```python
from build123d import *

# Parameters (mm, degrees)
ESQUISSE2_W             = 180
ESQUISSE2_H             = 90
BOSS_EXTRU_2_DEPTH      = 5
ESQUISSE3_W             = 170
ESQUISSE3_H             = 80
ESQUISSE3_W_2           = 160
ESQUISSE3_H_2           = 70
BOSS_EXTRU_3_DEPTH      = 30
ESQUISSE4_W             = 12
ESQUISSE4_H             = 13
ENL_V_MAT_EXTRU_1_DEPTH = 5


with BuildPart() as part:
    # Esquisse2 → Boss.-Extru.2 (new body)
    with BuildSketch(Plane.XY):
        with Locations((90, 45)):
            Rectangle(ESQUISSE2_W, ESQUISSE2_H)
    extrude(amount=BOSS_EXTRU_2_DEPTH)

    # Esquisse3 → Boss.-Extru.3 (add)
    with BuildSketch(Plane.XY.offset(5)):
        with Locations((90, 45)):
            Rectangle(ESQUISSE3_W, ESQUISSE3_H)
        with Locations((90, 45)):
            Rectangle(ESQUISSE3_W_2, ESQUISSE3_H_2, mode=Mode.SUBTRACT)
    extrude(amount=BOSS_EXTRU_3_DEPTH)

    # Esquisse4 → Enlèv. mat.-Extru.1 (cut)
    with BuildSketch(Plane(origin=(175, 0, 0), x_dir=(0, 0, -1), z_dir=(1, 0, 0))):
        with Locations((-13, 26.5)):
            Rectangle(ESQUISSE4_W, ESQUISSE4_H)
    extrude(amount=-ENL_V_MAT_EXTRU_1_DEPTH, mode=Mode.SUBTRACT)


solid = part.part
```
Can you work these out from the model? Positions are in its coordinate system, mm. A direction names the side the tool comes from. Coordinates: 2 decimals unless noted, no trailing zeros. Loops run counter-clockwise (first coordinate to the right, second up) from the corner with the lowest first, then second, coordinate; pieces in that order, holes last. Notation, with made-up numbers: (-26.5, -39.75) -> (19.5, -39.75) arc R27 ccw to (19.5, -21.75) -> close; hole circle Ø5 at (81, 36.25). An arc over 180 degrees is marked (long way). Answer as a JSON object with one key per item and string values.
1) If I drill on line 1 (X direction, y = 56, z = 17); line 2 (Y direction, x = 154, z = 29); line 3 (Z direction, x = 64.5, y = 46.5), over which ranges is the centre line in solid material (lowest first)?
Results:
{"line 1": "x = 5 to 10, 170 to 175", "line 2": "y = 5 to 10, 80 to 85", "line 3": "z = 0 to 5"}
2) Imagine slicing it at D-D (x = 35.5). Please give me the cut outline in (y, z).
Results:
{"outline": "(0, 0) -> (90, 0) -> (90, 5) -> (85, 5) -> (85, 35) -> (80, 35) -> (80, 5) -> (10, 5) -> (10, 35) -> (5, 35) -> (5, 5) -> (0, 5) -> close"}
3) Imagine slicing it at B-B (y = 30.5). Please give me the cut outline in (x, z), then the cut area to 3 significant figures.
Results:
{"outline": "(0, 0) -> (180, 0) -> (180, 5) -> (175, 5) -> (175, 7) -> (170, 7) -> (170, 5) -> (10, 5) -> (10, 35) -> (5, 35) -> (5, 5) -> (0, 5) -> close; (170, 19) -> (175, 19) -> (175, 35) -> (170, 35) -> close", "area": "1,140 mm^2"}
4) Imagine slicing it at C-C (y = 8). Please give me the cut outline in (x, z).
Results:
{"outline": "(0, 0) -> (180, 0) -> (180, 5) -> (175, 5) -> (175, 35) -> (5, 35) -> (5, 5) -> (0, 5) -> close"}
5) Imagine slicing it at A-A (z = 28). Please give me the cut outline in (x, y), then the cut area to 3 significant figures.
Results:
{"outline": "(5, 5) -> (175, 5) -> (175, 85) -> (5, 85) -> close; hole (10, 10) -> (170, 10) -> (170, 80) -> (10, 80) -> close", "area": "2,400 mm^2"}
6) For P1, Ø5, axis at y = 9.5, z = 6.5, coming from the -X side; P2, Ø6, axis at x = 96, z = 26, coming from the +Y side; P3, Ø9, axis at y = 58, z = 20, coming from the -X side; P4, Ø15, axis at x = 124.5, z = 14.5, coming from the -Y side, each with a flat end and sliding along its axis, tell me the tip position at first contact or that it passes through.
Results:
{"P1": "stops at x = 0", "P2": "stops at y = 85", "P3": "stops at x = 5", "P4": "stops at y = 5"}
7) Thinking about a two-plate mould opening in Y: for faces 1 (the face through (89, 5, 20)), 2 (the face through (173, 33, 13)), 3 (the face through (89, 90, 2)), which applies, pulls with the +Y half, pulls with the -Y half, needs draft (parallel to the pull), parting line crosses it, or undercut?
Results:
{"face 1": "pulls with the -Y half", "face 2": "undercut", "face 3": "pulls with the +Y half"}
8) For faces 4 (the face through (89, 80, 20)), 5 (the face through (89, 85, 20)), 6 (the face through (175, 44, 20)), which set-ups out of +Z, -Z, +X, -X, +Y, -Y let a thin tool reach every point of the face, with its end or its side?
Results:
{"face 4": "+Z", "face 5": "+Z, +X, -X, +Y", "face 6": "+Z, +X, +Y, -Y"}
